Input: part model. Units: mm. Frame: model coordinates. A direction names the side the tool comes from. Coordinates: 2 decimals unless noted, no trailing zeros. Order: outer loops, then holes, each group sorted by start corner. A loop starts at its lowest first (then second) coordinate and runs counter-clockwise, first axis right, second up. Notation, with made-up numbers: (-38.5, -16) - (-13.5, -16) arc R10 ccw to (-13.5, -11) - close; hole circle Ø1 at (87.25, 63). An arc over 180 degrees is marked (long way). Answer as CSV lines item,"result". Start each with the question number.
Item 1: Section B-B (z = 11). State how many separate pieces and enclosed holes the cut face has, and give its area (3 significant figures).
Item 2: Material intervals for line 1 along Y through (x, z) = (-39, 92.5); line 2 along Z through (x, y) = (0, 47.65); line 3 along Z through (x, y) = (-47.8, 31.75), sorted ascending.
Item 3: Access query for faces 1 (the cylindrical face through (-47, 22, 64)), 2 (the cylindrical face through (35.973, 37.859, 9.93)), 3 (the flat face through (-39.1, 37.8, 95)), 4 (the flat face through (16, 9.5, 1)). Directions: +Z, -Z, +X, -X, +Y, -Y. A direction counts if a zero-diameter tool reaches every point of the face in a straight line with its end or side. Return the directions, or none.
Item 4: Section C-C (x = 29). Output: boundary loops of the cut face in (y, z), and give its area (3 significant figures).
Item 5: Section A-A (x = 16.5). Output: boundary loops of the cut face in (y, z).
Item 6: First-contact query: pin 1 (2 mm diameter, centred on x = -23, y = 36.5, fed in from +Z); pin 2 (1 mm diameter, centred on x = 38, y = 36, fed in from +Z); pin 3 (1.5 mm diameter, centred on x = -24.5, y = -6, fed in from +Z). Flat tips, straight axial feed; report the tip coordinate or a pass-through.
from build123d import *

# Parameters (mm, degrees)
SKETCH_W                        = 100
SKETCH_H                        = 100
PAD_DEPTH                       = 100
SKETCH001_W                     = 90
SKETCH001_H                     = 90
POCKET_DEPTH                    = 95
POCKET001_DEPTH                 = 45
SKETCH003_R                     = 4
SKETCH003_R_2                   = 1
SKETCH003_R_3                   = 2.75
PAD001_DEPTH                    = 10
SKETCH004_W                     = 24
SKETCH004_H                     = 9
POCKET002_DEPTH                 = 5
SKETCH005_W                     = 5
SKETCH005_H                     = 10
POCKET003_DEPTH                 = 6
SKETCH006_W                     = 15
SKETCH006_H                     = 25
POCKET004_DEPTH                 = 3
SKETCH007_R                     = 1
POCKET005_DEPTH                 = 4
POCKET006_DEPTH                 = 6
POCKET006_LINEARPATTERN_2_DEPTH = 6
POCKET006_LINEARPATTERN_3_DEPTH = 6
POCKET006_LINEARPATTERN_4_DEPTH = 6
LINEARPATTERN001_COUNT          = 2
LINEARPATTERN001_PITCH          = 22
SKETCH009_R                     = 1
POCKET007_DEPTH                 = 4
SKETCH010_R                     = 1
POCKET008_DEPTH                 = 4
PAD002_DEPTH                    = 12
PAD002_MIRRORED001_2_DEPTH      = 12
LINEARPATTERN002_COUNT          = 2
LINEARPATTERN002_PITCH          = 78
SKETCH012_R                     = 1
POCKET009_DEPTH                 = 10
POCKET010_DEPTH                 = 20


with BuildPart() as part:
    # Sketch → Pad (new body)
    with BuildSketch(Plane.XY):
        Rectangle(SKETCH_W, SKETCH_H)
    extrude(amount=PAD_DEPTH)

    # Sketch001 (on Face6 of Pad) → Pocket (cut)
    with BuildSketch(Plane.XY.offset(100)):
        Rectangle(SKETCH001_W, SKETCH001_H)
    extrude(amount=-POCKET_DEPTH, mode=Mode.SUBTRACT)

    # Sketch002 → Pocket001 (cut)
    with BuildSketch(Plane.XZ):
        Polygon((28, 5), (48, 5), (48, 23), (28, 43), align=None)
    pocket001 = extrude(amount=-POCKET001_DEPTH, mode=Mode.SUBTRACT)

    # Mirrored: Pocket001 across XZ
    add(pocket001.mirror(Plane.XZ), mode=Mode.SUBTRACT)

    # Sketch003 (on Face11 of Mirrored) → Pad001 (join)
    with BuildSketch(Plane.XY.offset(5)):
        with Locations((-23, 36)):
            Circle(SKETCH003_R)
        with Locations((-23, 36)):
            Circle(SKETCH003_R_2, mode=Mode.SUBTRACT)
        with Locations((38, 36)):
            Circle(SKETCH003_R_3)
        with Locations((38, 36)):
            Circle(SKETCH003_R_2, mode=Mode.SUBTRACT)
        with Locations((44, -36)):
            Circle(SKETCH003_R_3)
        with Locations((44, -36)):
            Circle(SKETCH003_R_2, mode=Mode.SUBTRACT)
        with Locations((-23, -36)):
            Circle(SKETCH003_R_3)
        with Locations((-23, -36)):
            Circle(SKETCH003_R_2, mode=Mode.SUBTRACT)
    extrude(amount=PAD001_DEPTH)

    # Sketch004 (on Face23 of Pad001) → Pocket002 (cut)
    with BuildSketch(Plane(origin=(48, 0, 0), x_dir=(0, -1, 0), z_dir=(-1, 0, 0))):
        with Locations((17.5, 13.5)):
            Rectangle(SKETCH004_W, SKETCH004_H)
    extrude(amount=-POCKET002_DEPTH, mode=Mode.SUBTRACT)

    # Sketch005 (on Face16 of Pocket002) → Pocket003 (cut)
    with BuildSketch(Plane.XY.offset(5)):
        with Locations((16.5, -3)):
            Rectangle(SKETCH005_W, SKETCH005_H)
    extrude(amount=-POCKET003_DEPTH, mode=Mode.SUBTRACT)

    # Sketch006 (on Face4 of Pocket003) → Pocket004 (cut)
    with BuildSketch(Plane(origin=(0, 0, 0), x_dir=(1, 0, 0), z_dir=(0, 0, -1))):
        with Locations((16.5, 3)):
            Rectangle(SKETCH006_W, SKETCH006_H)
    extrude(amount=-POCKET004_DEPTH, mode=Mode.SUBTRACT)

    # Sketch007 (on Face15 of Pocket004) → Pocket005 (cut)
    with BuildSketch(Plane.YZ.offset(-45)):
        with Locations((-31.75, 62.25)):
            Circle(SKETCH007_R)
        with Locations((31.75, 62.25)):
            Circle(SKETCH007_R)
        with Locations((-31.75, 37.75)):
            Circle(SKETCH007_R)
        with Locations((31.75, 37.75)):
            Circle(SKETCH007_R)
    extrude(amount=-POCKET005_DEPTH, mode=Mode.SUBTRACT)

    # Sketch008 (on Face15 of Pocket005) → Pocket006 (cut)
    with BuildSketch(Plane.YZ.offset(-45)):
        with BuildLine():
            ThreePointArc((1.5, 62.5), (0, 64), (-1.5, 62.5))
            Line((-1.5, 62.5), (-1.5, 37.5))
            ThreePointArc((-1.5, 37.5), (0, 36), (1.5, 37.5))
            Line((1.5, 37.5), (1.5, 62.5))
        make_face()
    pocket006 = extrude(amount=-POCKET006_DEPTH, mode=Mode.SUBTRACT)

    # Sketch008 LinearPattern 2 → Pocket006 LinearPattern 2 (cut)
    with BuildSketch(Plane(origin=(-45, 7.333333, 0), x_dir=(0, 1, 0), z_dir=(1, 0, 0))):
        with BuildLine():
            ThreePointArc((1.5, 62.5), (0, 64), (-1.5, 62.5))
            Line((-1.5, 62.5), (-1.5, 37.5))
            ThreePointArc((-1.5, 37.5), (0, 36), (1.5, 37.5))
            Line((1.5, 37.5), (1.5, 62.5))
        make_face()
    pocket006_linearpattern_2 = extrude(amount=-POCKET006_LINEARPATTERN_2_DEPTH, mode=Mode.SUBTRACT)

    # Sketch008 LinearPattern 3 → Pocket006 LinearPattern 3 (cut)
    with BuildSketch(Plane(origin=(-45, 14.666667, 0), x_dir=(0, 1, 0), z_dir=(1, 0, 0))):
        with BuildLine():
            ThreePointArc((1.5, 62.5), (0, 64), (-1.5, 62.5))
            Line((-1.5, 62.5), (-1.5, 37.5))
            ThreePointArc((-1.5, 37.5), (0, 36), (1.5, 37.5))
            Line((1.5, 37.5), (1.5, 62.5))
        make_face()
    pocket006_linearpattern_3 = extrude(amount=-POCKET006_LINEARPATTERN_3_DEPTH, mode=Mode.SUBTRACT)

    # Sketch008 LinearPattern 4 → Pocket006 LinearPattern 4 (cut)
    with BuildSketch(Plane(origin=(-45, 22, 0), x_dir=(0, 1, 0), z_dir=(1, 0, 0))):
        with BuildLine():
            ThreePointArc((1.5, 62.5), (0, 64), (-1.5, 62.5))
            Line((-1.5, 62.5), (-1.5, 37.5))
            ThreePointArc((-1.5, 37.5), (0, 36), (1.5, 37.5))
            Line((1.5, 37.5), (1.5, 62.5))
        make_face()
    pocket006_linearpattern_4 = extrude(amount=-POCKET006_LINEARPATTERN_4_DEPTH, mode=Mode.SUBTRACT)

    # LinearPattern001: Pocket006, Pocket006 LinearPattern 2, Pocket006 LinearPattern 3, Pocket006 LinearPattern 4 ×2
    with Locations(*[(0, -i * LINEARPATTERN001_PITCH, 0) for i in range(1, LINEARPATTERN001_COUNT)]):
        add(pocket006, mode=Mode.SUBTRACT)
        add(pocket006_linearpattern_2, mode=Mode.SUBTRACT)
        add(pocket006_linearpattern_3, mode=Mode.SUBTRACT)
        add(pocket006_linearpattern_4, mode=Mode.SUBTRACT)

    # Sketch009 (on Face45 of MultiTransform) → Pocket007 (cut)
    with BuildSketch(Plane(origin=(45, 0, 0), x_dir=(0, -1, 0), z_dir=(-1, 0, 0))):
        with Locations((0, 80)):
            Circle(SKETCH009_R)
        with Locations((0, 35)):
            Circle(SKETCH009_R)
    extrude(amount=-POCKET007_DEPTH, mode=Mode.SUBTRACT)

    # Sketch010 (on Face46 of Pocket007) → Pocket008 (cut)
    with BuildSketch(Plane.XZ.offset(-45)):
        with Locations((0, 85)):
            Circle(SKETCH010_R)
        with Locations((0, 60)):
            Circle(SKETCH010_R)
    extrude(amount=-POCKET008_DEPTH, mode=Mode.SUBTRACT)

    # Sketch011 (on Face46 of Pocket008) → Pad002 (join)
    with BuildSketch(Plane.XZ.offset(-45)):
        Polygon((-45, 95), (-33, 95), (-33, 85), (-45, 73), align=None)
    pad002 = extrude(amount=PAD002_DEPTH)

    # Sketch011 Mirrored001 2 → Pad002 Mirrored001 2 (add)
    with BuildSketch(Plane(origin=(0, 45, 0), x_dir=(-1, 0, 0), z_dir=(0, 1, 0))):
        Polygon((-45, 95), (-33, 95), (-33, 85), (-45, 73), align=None)
    pad002_mirrored001_2 = extrude(amount=-PAD002_MIRRORED001_2_DEPTH)

    # LinearPattern002: Pad002, Pad002 Mirrored001 2 ×2
    with Locations(*[(0, -i * LINEARPATTERN002_PITCH, 0) for i in range(1, LINEARPATTERN002_COUNT)]):
        add(pad002)
        add(pad002_mirrored001_2)

    # Sketch012 (on Face55 of MultiTransform001) → Pocket009 (cut)
    with BuildSketch(Plane.XY.offset(95)):
        with Locations((-39, 39)):
            Circle(SKETCH012_R)
        with Locations((39, 39)):
            Circle(SKETCH012_R)
        with Locations((39, -39)):
            Circle(SKETCH012_R)
        with Locations((-39, -39)):
            Circle(SKETCH012_R)
    extrude(amount=-POCKET009_DEPTH, mode=Mode.SUBTRACT)

    # Sketch013 (on Face70 of Pocket009) → Pocket010 (cut)
    with BuildSketch(Plane.XY.offset(95)):
        Polygon((32, 42), (42, 32), (32, 32), align=None)
    extrude(amount=-POCKET010_DEPTH, mode=Mode.SUBTRACT)


solid = part.part
Determined:
1,separate pieces,"5"
1,enclosed holes,"4"
1,area,"1,690 mm^2"
2,line 1,"y = -50 to -40, -38 to -33, 33 to 38, 40 to 50"
2,line 2,"z = 0 to 59, 61 to 84, 86 to 100"
2,line 3,"z = 0 to 36.75, 38.75 to 61.25, 63.25 to 100"
3,face 1,"-X"
3,face 2,"none"
3,face 3,"+Z"
3,face 4,"-Z"
4,outline,"(-50, 0) - (50, 0) - (50, 100) - (45, 100) - (45, 5) - (-45, 5) - (-45, 100) - (-50, 100) - close"
4,area,"1,450 mm^2"
5,outline,"(-50, 0) - (-15.5, 0) - (-15.5, 3) - (-8, 3) - (-8, 5) - (-45, 5) - (-45, 100) - (-50, 100) - close; (2, 3) - (9.5, 3) - (9.5, 0) - (50, 0) - (50, 100) - (45, 100) - (45, 5) - (2, 5) - close"
6,pin 1,"stops at z = 15"
6,pin 2,"stops at z = 95"
6,pin 3,"stops at z = 5"
